Here's how the part is built. I have some questions about the finished solid (model axes, mm). Round coordinates to 2 decimals unless told otherwise and drop trailing zeros. Order: outer loops, then holes, each group sorted by start corner. A loop starts at its lowest first (then second) coordinate and runs counter-clockwise, first axis right, second up. Notation, with made-up numbers: (13.25, -14.75) -> (57.25, -14.75) arc R27 ccw to (57.25, 15.25) -> close; hole circle Ø6 at (53, 74.25). An arc over 180 degrees is marked (long way). One line per item, written item: value.
```python
from build123d import *

# Parameters (mm, degrees)
ESQUISSE1_W                    = 120
ESQUISSE1_H                    = 215
BOSS_EXTRU_1_DEPTH             = 6
ESQUISSE2_R                    = 1.6
ENL_V_MAT_EXTRU_1_DEPTH        = 138.798088748
R_P_TITION_LIN_AIRE1_OUTLINE_R = 1.6
R_P_TITION_LIN_AIRE1_DEPTH     = 6
ESQUISSE3_R                    = 4
ESQUISSE3_R_2                  = 5.5
ESQUISSE3_W                    = 15.409626965
ESQUISSE3_H                    = 38.248473635
ESQUISSE3_W_2                  = 15.900745579
ESQUISSE3_H_2                  = 26.603255198
ENL_V_MAT_EXTRU_2_DEPTH        = 138.798088748
ENL_V_MAT_EXTRU_3_DEPTH        = 138.798088748
ENL_V_MAT_EXTRU_4_DEPTH        = 138.798088748
ENL_V_MAT_EXTRU_4_DEPTH_BACK   = 138.798088748
ESQUISSE5_W                    = 60
ESQUISSE5_H                    = 33.99999972


# Read off the part's stored shape, not the designer's step: Répétition linéaire1
with BuildPart() as part:
    # Esquisse1 → Boss.-Extru.1 (new body)
    with BuildSketch(Plane.XY):
        with Locations((22.778700537, 2.5)):
            Rectangle(ESQUISSE1_W, ESQUISSE1_H)
    extrude(amount=BOSS_EXTRU_1_DEPTH)

    # Esquisse2 → Enlèv. mat.-Extru.1 (cut, through all)
    with BuildSketch(Plane.XY.offset(6)):
        with Locations((-27.221299463, -60)):
            Circle(ESQUISSE2_R)
    extrude(amount=-ENL_V_MAT_EXTRU_1_DEPTH, mode=Mode.SUBTRACT)

    # Répétition linéaire1 outline → Répétition linéaire1 (cut)
    with BuildSketch(Plane.XY):
        with Locations((-27.221299463, -10)):
            Circle(R_P_TITION_LIN_AIRE1_OUTLINE_R)
        with Locations((-22.221299463, 40)):
            Circle(R_P_TITION_LIN_AIRE1_OUTLINE_R)
        with Locations((-17.221299463, 90)):
            Circle(R_P_TITION_LIN_AIRE1_OUTLINE_R)
        with Locations((22.778700537, -60)):
            Circle(R_P_TITION_LIN_AIRE1_OUTLINE_R)
        with Locations((22.778700537, 15)):
            Circle(R_P_TITION_LIN_AIRE1_OUTLINE_R)
        with Locations((62.778700537, 90)):
            Circle(R_P_TITION_LIN_AIRE1_OUTLINE_R)
        with Locations((67.778700537, 40)):
            Circle(R_P_TITION_LIN_AIRE1_OUTLINE_R)
        with Locations((72.778700537, -10)):
            Circle(R_P_TITION_LIN_AIRE1_OUTLINE_R)
        with Locations((72.778700537, -60)):
            Circle(R_P_TITION_LIN_AIRE1_OUTLINE_R)
        with Locations((22.778700537, 90)):
            Circle(R_P_TITION_LIN_AIRE1_OUTLINE_R)
    extrude(amount=R_P_TITION_LIN_AIRE1_DEPTH, mode=Mode.SUBTRACT)

    # Esquisse3 → Enlèv. mat.-Extru.2 (cut, through all)
    with BuildSketch(Plane(origin=(0, 0, 0), x_dir=(-1, 0, 0), z_dir=(0, 0, -1))):
        with Locations((15.455236492, 68.53256443)):
            Circle(ESQUISSE3_R)
        with Locations((-32.238615261, 81.334914602)):
            Circle(ESQUISSE3_R_2)
        with Locations((-59.338617549, 81.334914602)):
            Circle(ESQUISSE3_R_2)
        with Locations((-45.804685817, 69.740615286)):
            Circle(ESQUISSE3_R_2)
        Polygon((-68.153753001, -58.054646), (-26.204418495, -58.054646), (-26.204418495, -14.671183794), (-30.693922011, -10.00000011), (-63.437167878, -10.00000011), (-68.153753001, -14.47508178), align=None)
        with Locations((13.783655533, -22.813946783)):
            Rectangle(ESQUISSE3_W, ESQUISSE3_H)
        with Locations((14.437094465, 21.783177691)):
            Rectangle(ESQUISSE3_W_2, ESQUISSE3_H_2)
        with BuildLine():
            Line((-30.778700537, -101), (-30.778700537, -105))
            Line((-30.778700537, -105), (-14.778700537, -105))
            Line((-14.778700537, -105), (-14.778700537, -101))
            ThreePointArc((-14.778700537, -101), (-22.778700537, -93), (-30.778700537, -101))
        make_face()
    extrude(amount=-ENL_V_MAT_EXTRU_2_DEPTH, mode=Mode.SUBTRACT)

    # Esquisse4 → Enlèv. mat.-Extru.3 (cut, through all)
    with BuildSketch(Plane.XY.offset(6)):
        Polygon((-37.221299463, 110), (-37.221299463, -5.00000078), (-25.60513741, 110), align=None)
        Polygon((71.162538485, 110), (82.778700537, 110), (82.778700537, -5.00000078), align=None)
    extrude(amount=-ENL_V_MAT_EXTRU_3_DEPTH, mode=Mode.SUBTRACT)

    # Esquisse5 → Enlèv. mat.-Extru.4 (cut, two sides: drawn at the far end of the back side and taken through both)
    with BuildSketch(Plane(origin=(0, 0, 0), x_dir=(-1, 0, 0), z_dir=(0, 0, -1)).offset(-ENL_V_MAT_EXTRU_4_DEPTH_BACK)):
        with Locations((-24.818757264, -88.00000014)):
            Rectangle(ESQUISSE5_W, ESQUISSE5_H)
    extrude(amount=ENL_V_MAT_EXTRU_4_DEPTH + ENL_V_MAT_EXTRU_4_DEPTH_BACK, mode=Mode.SUBTRACT)


solid = part.part
```
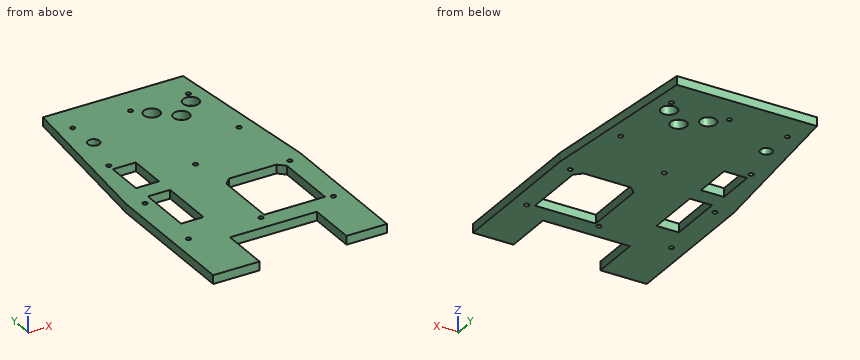
Q1. I want a section at B-B on z = 3.75. Give the number of separate pieces and of enclosed holes in the cut face, then the cut area to 3 significant figures.
Answers:
separate pieces: 1
enclosed holes: 18
area: 19,000 mm2
Q2. I want a section at A-A on x = -3. Write out the boundary of the cut face in (y, z).
Answers:
outline: (-71, 0) -> (110, 0) -> (110, 6) -> (-71, 6) -> close
Q3. I need wall thicknesses on line 1 along X through (y, z) = (-25, 3.75); line 2 along Y through (x, z) = (-20, 2); line 3 along X through (y, z) = (-6.5, 5.25). Which ranges of each line are inside material? Lowest first, please.
Answers:
line 1: -37.22 to -21.49, -6.08 to 26.2, 68.15 to 82.78
line 2: -105 to -41.94, -3.69 to 8.48, 35.08 to 110
line 3: -37.22 to -21.49, -6.08 to 82.78
Q4. For P1, Ø3, axis at y = 19.5, z = 3.5, coming from the +X side; P2, Ø1.9, axis at x = -22.22, y = 40, coming from the +Z side; P3, Ø3, axis at x = 23.5, z = 2.5, coming from the -Y side, each with a flat end and sliding along its axis, tell me the tip position at first contact or that it passes through.
Answers:
P1: x = 80.46
P2: through
P3: y = -71
Q5. I want a section at C-C on y = 47.5. Write out the boundary of the cut face in (x, z), then the cut area to 3 significant figures.
Answers:
outline: (-31.92, 0) -> (77.48, 0) -> (77.48, 6) -> (-31.92, 6) -> close
area: 656 mm2
